The model under review builds one solid part; all positions refer to its coordinate system, in mm. A direction names the side the tool comes from. Round coordinates to 2 decimals unless told otherwise and drop trailing zeros. Write each loop counter-clockwise with the first axis right and the second up, starting at its lowest first coordinate (ties: lowest second). Pieces come first, ordered by that corner, then holes. Notation, with made-up numbers: (40, -5) -> (65, -5) arc R30 ccw to (65, 28) -> close; hole circle Ø9 at (-17.5, 47.25). An arc over 180 degrees is marked (long way). Answer as a JSON object with one key per item and string values. Group by question number.
1) We need section C-C, the plane y = 101. Write out the cut boundary in (x, z), then the cut area to 3 significant figures.
2) Mouldability with a two-part tool opening along X and no side actions: class faces 3 (the flat face through (-10, 148, 312.5)), 4 (the flat face through (-10, 152, -300)), 5 (the cylindrical face through (1012.424, 147.9, -6.872)) as pulls with the +X half, pulls with the -X half, needs draft (parallel to the pull), parting line crosses it, or undercut.
3) To check wall thickness, follow probe 1 along Z at (x, y) = (712, 127.5); probe 2 along Z at (x, y) = (-405.5, 134.5); probe 3 along X at (y, z) = (285, -6). State the ranges of each line that lie inside material, in increasing order. Write a range as [from, to].
4) Insertion check: pin 1 Ø3 at (y, z) = (196, 30) entering from -X; pin 2 Ø8 at (y, z) = (125, 83.5) entering from +X; pin 3 Ø10 at (y, z) = (198, -54.5) entering from -X. Each pin has a flat end and moves straight along its axis. Give the tip position at first contact, or say it passes through.
5) We need section B-B, the plane z = 160.5. Write out the cut boundary in (x, y), then the cut area to 3 significant figures.
6) Machinability: for faces 1 (the flat face through (-5, 0, -302)), 2 (the cylindrical face through (-999.927, 152.1, -6.597)), which of the approach directions +Z, -Z, +X, -X, +Y, -Y give a long, thin tool a straight path to every point of the face, cutting with its end or side? Answer none if there is none.
7) We need section A-A, the plane x = 661. Write out the cut boundary in (y, z), then the cut area to 3 significant figures.
from build123d import *

# Parameters (mm, degrees)
SKIZZE3_W                       = 1400
SKIZZE3_H                       = 625
AUFSATZ_LINEAR_AUSTRAGEN1_DEPTH = 300
SKIZZE4_R                       = 312.5
AUFSATZ_LINEAR_AUSTRAGEN2_DEPTH = 300
SKIZZE5_W                       = 1400
SKIZZE5_H                       = 600
SCHNITT_LINEAR_AUSTRAGEN1_DEPTH = 1102.277667076
SKIZZE6_R                       = 300
SCHNITT_LINEAR_AUSTRAGEN2_DEPTH = 1102.277667076


with BuildPart() as part:
    # Skizze3 → Aufsatz-Linear austragen1 (new body)
    with BuildSketch(Plane(origin=(0, 0, 0), x_dir=(1, 0, 0), z_dir=(0, 1, 0))):
        Rectangle(SKIZZE3_W, SKIZZE3_H)
    extrude(amount=AUFSATZ_LINEAR_AUSTRAGEN1_DEPTH)

    # Skizze4 → Aufsatz-Linear austragen2 (add)
    with BuildSketch(Plane(origin=(0, 0, 0), x_dir=(1, 0, 0), z_dir=(0, 1, 0))):
        with Locations((-700, 0)):
            Circle(SKIZZE4_R)
    aufsatz_linear_austragen2 = extrude(amount=AUFSATZ_LINEAR_AUSTRAGEN2_DEPTH)

    # Spiegeln1: Aufsatz-Linear austragen2 across plane
    add(aufsatz_linear_austragen2.mirror(Plane(origin=(0, 0, 0), x_dir=(0, 0, 1), z_dir=(1, 0, 0))))

    # Skizze5 → Schnitt-Linear austragen1 (cut, through all)
    with BuildSketch(Plane(origin=(0, 300, 0), x_dir=(1, 0, 0), z_dir=(0, 1, 0))):
        Rectangle(SKIZZE5_W, SKIZZE5_H)
    extrude(amount=-SCHNITT_LINEAR_AUSTRAGEN1_DEPTH, mode=Mode.SUBTRACT)

    # Skizze6 → Schnitt-Linear austragen2 (cut, through all)
    with BuildSketch(Plane(origin=(0, 300, 0), x_dir=(1, 0, 0), z_dir=(0, 1, 0))):
        with Locations((-700, 0)):
            Circle(SKIZZE6_R)
    schnitt_linear_austragen2 = extrude(amount=-SCHNITT_LINEAR_AUSTRAGEN2_DEPTH, mode=Mode.SUBTRACT)

    # Spiegeln2: Schnitt-Linear austragen2 across plane
    add(schnitt_linear_austragen2.mirror(Plane(origin=(0, 0, 0), x_dir=(0, 0, 1), z_dir=(1, 0, 0))), mode=Mode.SUBTRACT)


solid = part.part
Here are the results:
{
 "1": {"outline": "(-700, -312.5) -> (700, -312.5) arc R312.5 ccw to (700, 312.5) -> (-700, 312.5) arc R312.5 ccw to start; hole (-700, -300) -> (700, -300) arc R300 ccw to (700, 300) -> (-700, 300) arc R300 ccw to start", "area": "59,100 mm^2"},
 "2": {"face 3": "needs draft", "face 4": "undercut", "face 5": "pulls with the +X half"},
 "3": {"probe 1": "z = [-312.27, -299.76], [299.76, 312.27]", "probe 2": "z = [-312.5, -300], [300, 312.5]", "probe 3": "x = [-1012.44, -999.94], [999.94, 1012.44]"},
 "4": {"pin 1": "stops at x = -1011.2", "pin 2": "stops at x = 1002.22", "pin 3": "stops at x = -1008.55"},
 "5": {"outline": "(-968.13, 0) -> (-953.46, 0) -> (-953.46, 300) -> (-968.13, 300) -> close; (953.46, 0) -> (968.13, 0) -> (968.13, 300) -> (953.46, 300) -> close", "area": "8,810 mm^2"},
 "6": {"face 1": "+Z, -Z, +X, -X, -Y", "face 2": "+Y, -Y"},
 "7": {"outline": "(0, -312.5) -> (300, -312.5) -> (300, -300) -> (0, -300) -> close; (0, 300) -> (300, 300) -> (300, 312.5) -> (0, 312.5) -> close", "area": "7,500 mm^2"}
}
